Input: part model. Units: mm. Frame: model coordinates. A direction names the side the tool comes from. Coordinates: 2 decimals unless noted, no trailing zeros. Order: outer loops, then holes, each group sorted by start corner. A loop starts at its lowest first (then second) coordinate and runs counter-clockwise, first axis right, second up.
from build123d import *
from OCP.BRepFilletAPI import BRepFilletAPI_MakeChamfer

# Parameters (mm, degrees)
BOSS_EXTRUDE1_DEPTH = 80
CUT_EXTRUDE2_DEPTH  = 82.280481137
SKETCH6_W           = 4
SKETCH6_H           = 13
BOSS_EXTRUDE6_DEPTH = 70
BOSS_EXTRUDE7_REACH = 148.366
BOSS_EXTRUDE8_REACH = 152.403
CUT_EXTRUDE3_DEPTH  = 146.557626962
CUT_EXTRUDE4_DEPTH  = 142.8119282
CHAMFER3_START      = -30
CHAMFER3_OUTLINE_W  = 24
CHAMFER3_OUTLINE_H  = 27
CHAMFER3_DEPTH      = 4.140431355
CHAMFER4_START      = -11
CHAMFER4_OUTLINE_W  = 75
CHAMFER4_OUTLINE_H  = 14
CHAMFER4_DEPTH      = 2.728063486
CHAMFER5_START      = -38
CHAMFER5_OUTLINE_W  = 21
CHAMFER5_OUTLINE_H  = 26
CHAMFER5_DEPTH      = 3.409757195
CHAMFER7_SIZE       = 3
CHAMFER7_SIZE2      = 3.268453219
CHAMFER8_START      = -40
CHAMFER8_DEPTH      = 3.210737533
SKETCH20_W          = 40
SKETCH20_H          = 40
CUT_EXTRUDE5_DEPTH  = 103.734976835


with BuildPart() as part:
    # Sketch1 → Boss-Extrude1 (new body)
    with BuildSketch(Plane(origin=(0, 0, 0), x_dir=(1, 0, 0), z_dir=(0, 1, 0))):
        Polygon((3.622068507, 4.197822071), (3.622068507, -8.802177929), (-0.377931493, -8.802177929), (-0.377931493, 4.197822071), (-3.677931493, 4.197822071), (-3.677931493, -8.802177929), (-7.677931493, -8.802177929), (-7.677931493, 8.878435326), align=None)
    extrude(amount=BOSS_EXTRUDE1_DEPTH)

    # Sketch2 → Cut-Extrude2 (cut, through all)
    with BuildSketch(Plane.ZY.offset(7.677931493)):
        Polygon((8.802177929, 80), (-8.878435326, 80), (-8.878435326, 72.676450199), align=None)
    extrude(amount=-CUT_EXTRUDE2_DEPTH, mode=Mode.SUBTRACT)

    # Sketch6 → Boss-Extrude6 (add, along a direction that is not the sketch's normal)
    with BuildSketch(Plane.XY.offset(8.802177929)):
        with Locations((-5.677931493, 73.5)):
            Rectangle(SKETCH6_W, SKETCH6_H)
        with Locations((1.622068507, 73.5)):
            Rectangle(SKETCH6_W, SKETCH6_H)
    extrude(amount=BOSS_EXTRUDE6_DEPTH, dir=(0, 0.3826834323650841, 0.9238795325112892))

    # Boss-Extrude7: up to this plane
    boss_extrude7_end = Plane(origin=(3.622068507, 80, -4.197822071), z_dir=(-0.3826834323650841, 0, 0.9238795325112892))
    # Sketch7 → Boss-Extrude7 (add, up to the surface)
    with BuildSketch(Plane.XY.offset(73.473745205), mode=Mode.PRIVATE) as boss_extrude7_sk1:
        Polygon((-7.677931493, 106.787840266), (3.622068507, 106.787840266), (-7.677931493, 111.46845352), align=None)
    boss_extrude7_tool1 = split(extrude(boss_extrude7_sk1.sketch, amount=BOSS_EXTRUDE7_REACH, dir=(0, -0.382683432365, -0.923879532511), mode=Mode.PRIVATE), bisect_by=boss_extrude7_end, keep=Keep.BOTH, mode=Mode.PRIVATE)
    add(boss_extrude7_tool1.solids().sort_by_distance((-3.911265, 108.348045, 73.473745))[0])

    # Boss-Extrude8: up to this plane
    boss_extrude8_end = Plane(origin=(3.622068507, 80, -4.197822071), z_dir=(-0.3826834323650841, 0, 0.9238795325112892))
    # Sketch16 → Boss-Extrude8 (add, up to the surface)
    with BuildSketch(Plane.XY.offset(73.473745205), mode=Mode.PRIVATE) as boss_extrude8_sk1:
        Polygon((3.622068507, 106.787840266), (12.814456663, 115.980228421), (9.986029538, 118.808655546), (0.793641383, 109.61626739), (-1.539810995, 111.949719768), (7.65257716, 121.142107924), (4.824150035, 123.970535048), (-7.677931493, 111.46845352), align=None)
    boss_extrude8_tool1 = split(extrude(boss_extrude8_sk1.sketch, amount=BOSS_EXTRUDE8_REACH, dir=(0, -0.382683432365, -0.923879532511), mode=Mode.PRIVATE), bisect_by=boss_extrude8_end, keep=Keep.BOTH, mode=Mode.PRIVATE)
    add(boss_extrude8_tool1.solids().sort_by_distance((8.029162, 111.573135, 73.473745))[0])

    # Sketch17 → Cut-Extrude3 (cut, through all)
    with BuildSketch(Plane.ZY.offset(7.677931493)):
        Polygon((73.473745205, 93.787840266), (58.313175353, 130.388693616), (73.473745205, 136.668407262), align=None)
    extrude(amount=-CUT_EXTRUDE3_DEPTH, mode=Mode.SUBTRACT)

    # Sketch19 → Cut-Extrude4 (cut, through all)
    with BuildSketch(Plane.ZY.offset(7.677931493)):
        Polygon((73.473745205, 93.787840266), (19.545714219, 71.450118439), (5.092625448, 106.342961367), (59.020656435, 128.680683193), align=None)
    extrude(amount=-CUT_EXTRUDE4_DEPTH, mode=Mode.SUBTRACT)

    # Mirror9: part across plane


with BuildPart() as part_1:
    add(part.part)
    add(part.part.mirror(Plane(origin=(2.014593878, 0, -4.863659863), x_dir=(0.9238795325112891, 0, 0.3826834323650842), z_dir=(0.3826834323650841, 0, -0.9238795325112892))))

    # Chamfer3: read off the stored shape, not the designer's step
    # Chamfer3 outline → Chamfer3 (cut)
    with BuildSketch(Plane(origin=(0, 0, 0), x_dir=(0.4459030144065531, 0.4972805165228299, -0.7442328866893325), z_dir=(0.8950812821990801, -0.24773044161799307, 0.3707548065131521)).offset(CHAMFER3_START)):
        with Locations((45, 59.5)):
            Rectangle(CHAMFER3_OUTLINE_W, CHAMFER3_OUTLINE_H)
    extrude(amount=CHAMFER3_DEPTH, mode=Mode.SUBTRACT)

    # Chamfer4: read off the stored shape, not the designer's step
    # Chamfer4 outline → Chamfer4 (cut)
    with BuildSketch(Plane(origin=(0, 0, 0), x_dir=(0, 1, 0), z_dir=(0.9238795325112892, 0, 0.3826834323650841)).offset(CHAMFER4_START)):
        with Locations((36.5, -5)):
            Rectangle(CHAMFER4_OUTLINE_W, CHAMFER4_OUTLINE_H)
    extrude(amount=CHAMFER4_DEPTH, mode=Mode.SUBTRACT)

    # Chamfer5: read off the stored shape, not the designer's step
    # Chamfer5 outline → Chamfer5 (cut)
    with BuildSketch(Plane(origin=(0, 0, 0), x_dir=(0.3652745046018862, 0.9288881868246626, 0.061165943673236425), z_dir=(0.9161327263409628, -0.37036027915745895, 0.15340825059130198)).offset(CHAMFER5_START)):
        with Locations((74.5, 5)):
            Rectangle(CHAMFER5_OUTLINE_W, CHAMFER5_OUTLINE_H)
    extrude(amount=CHAMFER5_DEPTH, mode=Mode.SUBTRACT)

    # Chamfer7: one chamfer whose edges measure the first distance from different faces: ONE call of the kernel's chamfer builder (chamfer() names one face for all edges)
    chamfer7_edges_1 = [part_1.edges().sort_by_distance(p)[0] for p in [
        (-7.677931493, 69.225059219, 14.173946074),
        (8.622563718, 69.225059219, -25.178930536),
        (4.824150035, 33.5, -21.380516854),
        (-7.677931493, 33.5, 8.802177929),
    ]]
    chamfer7_edges_2 = [part_1.edges().sort_by_distance(p)[0] for p in [
        (9.269880183, 94.608411482, -8.145633747),
        (4.824150035, 94.608411482, 2.587308271),
    ]]
    chamfer7_side_2 = [part_1.faces().sort_by_distance(p)[0] for p in [
        (3.501171082, 89.374799079, -6.853796043),
    ]]
    chamfer7 = BRepFilletAPI_MakeChamfer(part_1.part.solid().wrapped)
    for e in chamfer7_edges_1:
        chamfer7.Add(CHAMFER7_SIZE, e.wrapped)
    for e in chamfer7_edges_2:
        chamfer7.Add(CHAMFER7_SIZE, CHAMFER7_SIZE2, e.wrapped, chamfer7_side_2[0].wrapped)  # the first distance lies on this face
    add(Compound.cast(chamfer7.Shape()), mode=Mode.REPLACE)

    # Chamfer8: read off the stored shape, not the designer's step
    # Chamfer8 outline → Chamfer8 (cut)
    with BuildSketch(Plane(origin=(0, 0, 0), x_dir=(0.6542484614665716, 0.42811862617005, -0.6234367590982206), z_dir=(0.7562796775456972, -0.37036027915745917, 0.5393276489795283)).offset(CHAMFER8_START)):
        Polygon((57.189510074, 50), (58.060381385, 66), (36, 66), (36, 50), align=None)
    extrude(amount=CHAMFER8_DEPTH, mode=Mode.SUBTRACT)

    # Sketch20 → Cut-Extrude5 (cut, through all)
    with BuildSketch(Plane(origin=(-7.642272839, 0, -3.165533057), x_dir=(-0.3826834323650836, 0, 0.9238795325112894), z_dir=(-0.9238795325112893, 0, -0.38268343236508356))):
        with Locations((-6.292508137, 20)):
            Rectangle(SKETCH20_W, SKETCH20_H)
    extrude(amount=-CUT_EXTRUDE5_DEPTH, mode=Mode.SUBTRACT)


solid = part_1.part
Item 1: Access query for faces 5 (the face through (11.42, 53.311, -14.785)), 6 (the face through (11.44, 89.06, 5.16)), 7 (the face through (-6.16, 54.3, 7.32)). Directions: +Z, -Z, +X, -X, +Y, -Y. A direction counts if a zero-diameter tool reaches every point of the face in a straight line with its end or side. Return the directions, or none.
Response values:
face 5: -Z, +X, -Y
face 6: +X, +Y
face 7: +Z, -X, -Y
Item 2: Cut plane C-C on x = 8.5. Return loops of the section in (y, z), then the cut area to 3 significant figures.
Response values:
outline: (40, -14.73) - (79.13, -14.73) - (80.5, -19.4) - (67.5, -19.4) - (67.91, -20.81) - (72.4, -25.06) - (80.2, -25.06) - (89.47, -18.69) - (92.87, -10.49) - (90.76, -3.98) - (90.16, -3.38) - (84.77, -16.38) - (81.47, -13.08) - (91.54, 11.22) - (86.71, 13.22) - (77.47, -9.08) - (40, -9.08) - close
area: 535 mm2
Item 3: Ray query, probe 1 along X at (y, z) = (86, 10); probe 2 along Z at (x, y) = (11.5, 70); probe 3 along X at (y, z) = (46.5, -13). Return the intervals inside material, ascending.
Response values:
probe 1: x = -4.66 to -1.2, 3.47 to 9.13
probe 2: z = -24.13 to -22.4, -17.73 to -12.08
probe 3: x = -3.56 to 2.1, 6.77 to 12.42
Item 4: Cut plane A-A on y = 91.5. Return loops of the section in (x, z).
Response values:
outline: (-1.87, 11.24) - (2.62, 0.4) - (7.22, 0.88) - (7.65, 1.91) - (3.79, 11.24) - close; (6.17, -8.16) - (10.66, -19) - (14.66, -15) - (10.79, -5.67) - (9.76, -5.24) - close; (8.46, 11.24) - (9.99, 7.54) - (11.52, 11.24) - close; (16.43, -8) - (17.96, -11.7) - (20.12, -9.53) - close
Item 5: Cut plane D-D on y = 58. Return loops of the section in (x, z), then the cut area to 3 significant figures.
Response values:
outline: (-7.68, -3.08) - (-3.58, -12.98) - (2.7, -19.26) - (6.95, -19.26) - (7.65, -18.55) - (-1.54, -9.36) - (0.79, -7.03) - (9.99, -16.22) - (12.81, -13.39) - (3.62, -4.2) - (3.62, 8.8) - (-0.38, 8.8) - (-0.38, -4.2) - (-3.68, -4.2) - (-3.68, 8.8) - (-4.68, 8.8) - (-7.68, 5.8) - close
area: 240 mm2
Item 6: Draft query along Z for faces 1 (the face through (1.594, 69.194, 14.099)), 2 (the face through (6.599, 81.927, -12.742)), 3 (the face through (-0.32, 81.93, 3.95)), 4 (the face through (3.42, 81.94, -16.74)). Return one class per face: pulls with the +Z half, pulls with the -Z half, needs draft (parallel to the pull), parting line crosses it, or undercut.
Response values:
face 1: pulls with the +Z half
face 2: undercut
face 3: undercut
face 4: pulls with the -Z half
Item 7: Pin query (flat end, axial travel): pin 1 Ø2 at (y, z) = (83, 0.5) entering from -X; pin 2 Ø3.5 at (x, y) = (6, 58) entering from -Z; pin 3 Ø1.2 at (x, y) = (2.5, 58.5) entering from +Z. Return the tip coordinate at first contact, or that it passes through.
Response values:
pin 1: stops at x = -4.72
pin 2: stops at z = -19.26
pin 3: stops at z = 8.8
Item 8: Cut plane B-B on z = 4. Return loops of the section in (x, y).
Response values:
outline: (-7.68, 40) - (-3.68, 40) - (-3.68, 78.01) - (-0.38, 78.01) - (-0.38, 40) - (3.62, 40) - (3.62, 78.01) - (12.81, 87.2) - (9.99, 90.03) - (0.79, 80.84) - (-1.54, 83.17) - (7.65, 92.37) - (7.22, 92.79) - (2.62, 92.99) - (-3.18, 87.19) - (-7.68, 76.06) - close
